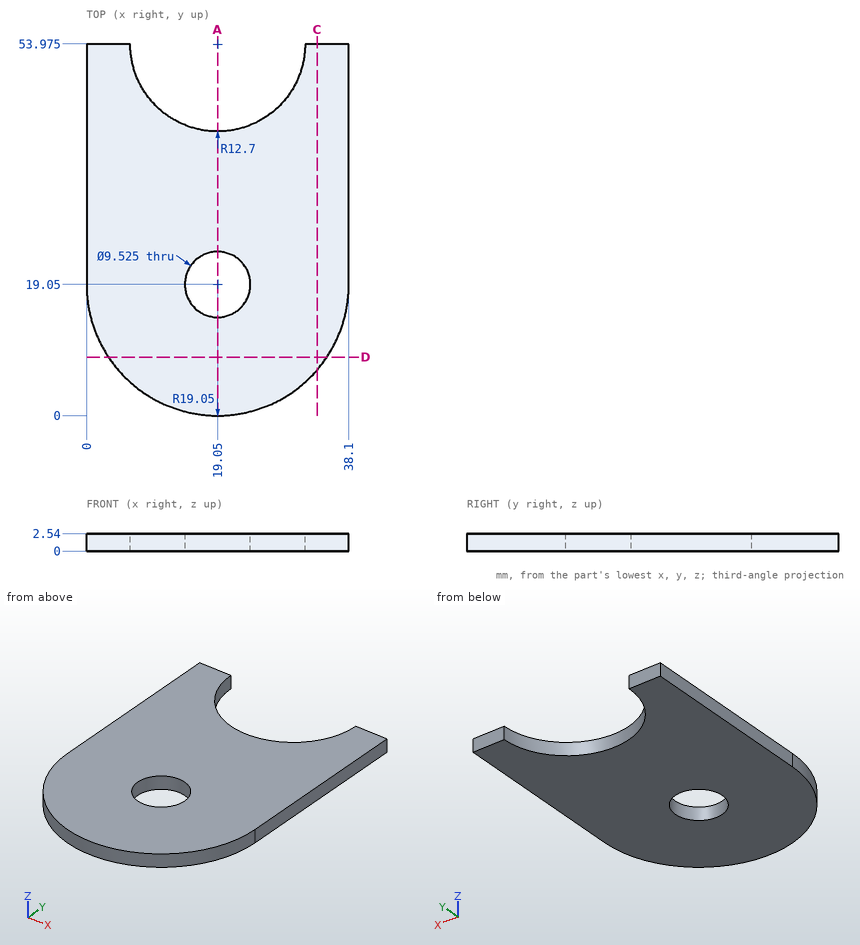
Study the drawing (mm; zero at the part's minimum x, y, z) and answer. Round coordinates to 2 decimals unless told otherwise and drop trailing zeros. Write each loop counter-clockwise with the first axis right and the second up, starting at its lowest first coordinate (ties: lowest second). Pieces come first, ordered by that corner, then holes. Notation, with made-up numbers: (46, 33) - (88, 33) arc R37 cw to (88, 69) - close; hole circle Ø7 at (-35, 84.5). An arc over 180 degrees is marked (long way). Use a Markdown table: item, result. Add a question column.
1. The part is cut by section C-C (x = 33.5). Write down the section's boundary in (y, z) (3 decimals), and give its area (3 significant figures).
2. Flat-ended cylindrical pins translate along their axes: P1, Ø1, axis at y = 11.5, z = 1.5, coming from the +X side; P2, Ø4, axis at x = 18, y = 17.5, coming from the -Z side. Find the tip coordinate at first contact, or state that the pin passes through.
3. The part is cut by section D-D (y = 8.5). Write down the section's boundary in (x, z).
4. Consider line 1 (Y direction, x = 19.05, z = 0.6) (1 decimal); line 2 (X direction, y = 49.5, z = 0.55); line 3 (X direction, y = 15, z = 0.65). Determine where each line is inside the solid, lowest interval first.
5. The part is cut by section A-A (x = 19.05). Write down the section's boundary in (y, z) (1 decimal).
Reported:
| question | item | result |
|---|---|---|
| 1 | outline | (6.636, 0) - (53.975, 0) - (53.975, 2.54) - (6.636, 2.54) - close |
| 1 | area | 120 mm^2 |
| 2 | P1 | x = 36.75 |
| 2 | P2 | through |
| 3 | outline | (3.19, 0) - (34.91, 0) - (34.91, 2.54) - (3.19, 2.54) - close |
| 4 | line 1 | 0 to 14.3, 23.8 to 41.3 |
| 4 | line 2 | 0 to 7.16, 30.94 to 38.1 |
| 4 | line 3 | 0.44 to 16.54, 21.56 to 37.66 |
| 5 | outline | (0, 0) - (14.3, 0) - (14.3, 2.5) - (0, 2.5) - close; (23.8, 0) - (41.3, 0) - (41.3, 2.5) - (23.8, 2.5) - close |
